The model under review builds one solid part; all positions refer to its coordinate system, in mm. A direction names the side the tool comes from. Round coordinates to 2 decimals unless told otherwise and drop trailing zeros. Order: outer loops, then holes, each group sorted by start corner. A loop starts at its lowest first (then second) coordinate and runs counter-clockwise, first axis right, second up. Notation, with made-up numbers: (14.25, 63) -> (39.25, 63) arc R11 ccw to (39.25, 83) -> close; hole circle Ø5 at (-6, -19). An arc over 180 degrees is marked (long way). Return JSON: item names as keys, results as strings. Group by question number.
from build123d import *

# Parameters (mm, degrees)
F0_W     = 9.525
F0_H     = 9.525
F0_R     = 2.38125
F1_DEPTH = 4.7625
F2_R     = 5.08
F3_R     = 3.175


with BuildPart() as f1:
    # F0 (on Top) → F1 (new body)
    with BuildSketch(Plane.XY):
        with BuildLine():
            ThreePointArc((-6.35, -6.35), (0, 0), (-6.35, 6.35))
            Line((-6.35, 6.35), (-69.85, 6.35))
            Line((-69.85, 6.35), (-79.375, 9.5377))
            Line((-79.375, 9.5377), (-98.4504, 9.5377))
            Line((-98.4504, 9.5377), (-98.4504, -9.5377))
            Line((-98.4504, -9.5377), (-79.375, -9.5377))
            Line((-79.375, -9.5377), (-69.85, -6.35))
            Line((-69.85, -6.35), (-6.35, -6.35))
        make_face()
        with Locations((-88.9127, 0)):
            Rectangle(F0_W, F0_H, mode=Mode.SUBTRACT)
        with Locations((-63.5, 0)):
            Circle(F0_R, mode=Mode.SUBTRACT)
        with Locations((-19.05, 0)):
            Circle(F0_R, mode=Mode.SUBTRACT)
    extrude(amount=F1_DEPTH)

    # F2
    f2_edges = [f1.edges().sort_by_distance(p)[0] for p in [
        (-98.4504, 9.5377, 2.38125),
        (-98.4504, -9.5377, 2.38125),
    ]]
    fillet(f2_edges, radius=F2_R)

    # F3
    f3_edges = [f1.edges().sort_by_distance(p)[0] for p in [
        (-84.1502, -4.7625, 2.38125),
        (-84.1502, 4.7625, 2.38125),
        (-93.6752, 4.7625, 2.38125),
        (-93.6752, -4.7625, 2.38125),
    ]]
    fillet(f3_edges, radius=F3_R)


solid = f1.part
Item 1: Consider section B-B on x = -19.05. State the section outline as (y, z) points, plus the area to 3 significant figures.
Item 2: Insertion check: pin 1 Ø1.4 at (x, z) = (-46, 3.5) entering from +Y; pin 2 Ø5 at (x, y) = (-53.5, -2) entering from -Z; pin 3 Ø4 at (x, y) = (-86.5, 0.5) entering from -Z. Each pin has a flat end and moves straight along its axis. Give the tip position at first contact, or say it passes through.
Item 3: Consider section A-A on y = 0. State the section outline as (x, z) points.
Item 4: For faces 1 (the face through (-86, -9.538, 2)), 2 (the face through (0, 0, 2)), 3 (the face through (-39, -6.35, 2)), 4 (the face through (-38, 6.35, 2)), 5 (the face through (-89, 4.762, 2)), list the 3-axis set-ups (+Z, -Z, +X, -X, +Y, -Y) from which the entire face can be reached by the end or side of a thin tool; tool diameter is ignored.
Item 5: The part is to be moulded in two halves that separate along Y. For faces 6 (the face through (-86, 9.538, 2)), 7 (the face through (-96.92, -8.09, 2.41)), 8 (the face through (-21.43, 0.1, 2.35)), say which applies: +Y half, -Y half, draft (parallel to the pull), parting line (faces both ways), or undercut.
Item 6: Wall thickness on line 1 along Y through (x, z) = (-19.05, 1.75); line 2 along X through (y, z) = (1.5, 4.4): over which ranges is each line inside the solid? List them lowest first.
Item 7: Consider section D-D on x = -42.5. State the section outline as (y, z) points.
Item 8: Consider section C-C on z = 0.8. Give the number of separate pieces and of enclosed holes in the cut face, plus the area to 3 significant figures.
Values:
{
 "1": {"outline": "(-6.35, 0) -> (-2.38, 0) -> (-2.38, 4.76) -> (-6.35, 4.76) -> close; (2.38, 0) -> (6.35, 0) -> (6.35, 4.76) -> (2.38, 4.76) -> close", "area": "37.8 mm^2"},
 "2": {"pin 1": "y = 6.35", "pin 2": "z = 0", "pin 3": "through"},
 "3": {"outline": "(-98.45, 0) -> (-93.68, 0) -> (-93.68, 4.76) -> (-98.45, 4.76) -> close; (-84.15, 0) -> (-65.88, 0) -> (-65.88, 4.76) -> (-84.15, 4.76) -> close; (-61.12, 0) -> (-21.43, 0) -> (-21.43, 4.76) -> (-61.12, 4.76) -> close; (-16.67, 0) -> (0, 0) -> (0, 4.76) -> (-16.67, 4.76) -> close"},
 "4": {"face 1": "+Z, -Z, +X, -X, -Y", "face 2": "+Z, -Z, +X", "face 3": "+Z, -Z, +X, -Y", "face 4": "+Z, -Z, +X, +Y", "face 5": "+Z, -Z"},
 "5": {"face 6": "+Y half", "face 7": "-Y half", "face 8": "undercut"},
 "6": {"line 1": "-6.35 to -2.38, 2.38 to 6.35", "line 2": "-98.45 to -93.68, -84.15 to -65.35, -61.65 to -20.9, -17.2 to -0.18"},
 "7": {"outline": "(-6.35, 0) -> (6.35, 0) -> (6.35, 4.76) -> (-6.35, 4.76) -> close"},
 "8": {"separate pieces": "1", "enclosed holes": "3", "area": "1,260 mm^2"}
}
